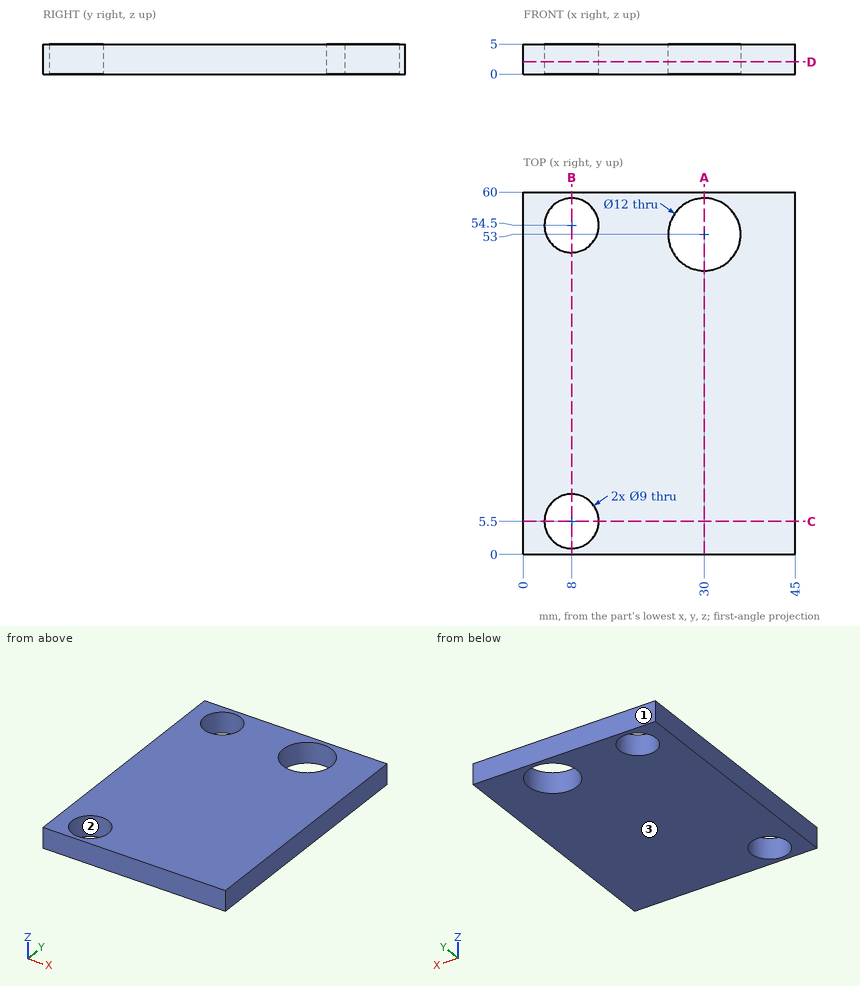
Could you check a few things on this drawing? It's one solid part, dimensions in mm from its lowest x, y, z. Round coordinates to 2 decimals unless told otherwise and drop trailing zeros. Loops run counter-clockwise (first coordinate to the right, second up) from the corner with the lowest first, then second, coordinate; pieces in that order, holes last. Notation, with made-up numbers: (3, -34.75) -> (36, -34.75) arc R31 ccw to (36, -9.75) -> close; hole circle Ø11 at (58.5, 2). An arc over 180 degrees is marked (long way). Write each question's results on one line, items separated by ' | '.
(1) For P1, Ø7, axis at x = 8, y = 5.5, coming from the +Z side; P2, Ø1.5, axis at x = 11.5, y = 37, coming from the -Z side, each with a flat end and sliding along its axis, tell me the tip position at first contact or that it passes through.
Worked answers:
P1: through | P2: z = 0
(2) We'd pull the mould along Y, two halves only. Please class the marked faces 1, 2 and 3: released by +Y, released by -Y, zero draft, split by the parting line, or undercut.
Worked answers:
face 1: released by +Y | face 2: undercut | face 3: zero draft
(3) If I drill on L1, parallel to Y at x = 8, z = 1.6; L2, parallel to Y at x = 30, z = 3.85; L3, parallel to Y at x = 12, z = 1.6, over which ranges is the centre line in solid material (lowest first)?
Worked answers:
L1: 0 to 1, 10 to 50, 59 to 60 | L2: 0 to 47, 59 to 60 | L3: 0 to 3.44, 7.56 to 52.44, 56.56 to 60
(4) If we section it at A-A, the plane x = 30: List the corners of the cut face in (y, z) for me, then the cut area to 3 significant figures.
Worked answers:
outline: (0, 0) -> (47, 0) -> (47, 5) -> (0, 5) -> close; (59, 0) -> (60, 0) -> (60, 5) -> (59, 5) -> close | area: 240 mm2
(5) If we section it at D-D, the plane z = 2.05: List the corners of the cut face in (x, y) for me.
Worked answers:
outline: (0, 0) -> (45, 0) -> (45, 60) -> (0, 60) -> close; hole circle Ø9 at (8, 5.5); hole circle Ø9 at (8, 54.5); hole circle Ø12 at (30, 53)
(6) If we section it at B-B, the plane x = 8: List the corners of the cut face in (y, z) for me, then the cut area to 3 significant figures.
Worked answers:
outline: (0, 0) -> (1, 0) -> (1, 5) -> (0, 5) -> close; (10, 0) -> (50, 0) -> (50, 5) -> (10, 5) -> close; (59, 0) -> (60, 0) -> (60, 5) -> (59, 5) -> close | area: 210 mm2
(7) If we section it at C-C, the plane y = 5.5: List the corners of the cut face in (x, z) for me, then the cut area to 3 significant figures.
Worked answers:
outline: (0, 0) -> (3.5, 0) -> (3.5, 5) -> (0, 5) -> close; (12.5, 0) -> (45, 0) -> (45, 5) -> (12.5, 5) -> close | area: 180 mm2
